The drawing under review shows one solid part. Ordinate dimensions are in mm from its lowest x, y, z. A direction names the side the tool comes from. Give positions to 0.01 mm unless a question says otherwise; leave off trailing zeros. Order: outer loops, then holes, each group sorted by start corner. A loop starts at its lowest first (then second) coordinate and runs counter-clockwise, first axis right, second up. Notation, with made-up numbers: (11.25, 24.5) -> (61.25, 24.5) arc R10 cw to (61.25, 40.5) -> close; hole circle Ø3 at (8.25, -24.5). An arc over 180 degrees is marked (long way). One line per item, written item: value. Start each with the question number.
1) Consider section C-C (z = 12). State the section outline as (x, y) points, plus the area to 3 significant figures.
2) Tool access review of the marked faces 1, 2 and 3: name each direction out of +Z, -Z, +X, -X, +Y, -Y from which nothing blocks a thin tool from reaching the whole face with its end or side.
3) The part is to be moulded in two halves that separate along Y. For the marked faces 4, 5, 6 and 7, say which applies: released by +Y, released by -Y, zero draft, split by the parting line, or undercut.
4) For pin 1 (5 mm diameter, centred on x = 8, y = 6, fed in from -Z); pin 2 (0.9 mm diameter, centred on x = 8.5, z = 4.5, fed in from +Y); pin 3 (1.5 mm diameter, centred on x = 7, y = 28, fed in from +Z), all flat-tipped, find the tip position at first contact; note any pin that passes through.
5) Consider section A-A (x = 10.5). State how many separate pieces and enclosed holes the cut face has, plus the area to 3 significant figures.
6) Wall thickness on line 1 along Z through (x, y) = (6, 14.9); line 2 along Z through (x, y) = (10.5, 24); line 3 along Y through (x, z) = (5.25, 3.5): over which ranges is each line inside the solid? List them lowest first. Write a range as from..to.
7) Consider section B-B (y = 14.9). State the section outline as (x, z) points.
8) Consider section D-D (y = 3.75). State the section outline as (x, z) points, plus the area to 3 significant figures.
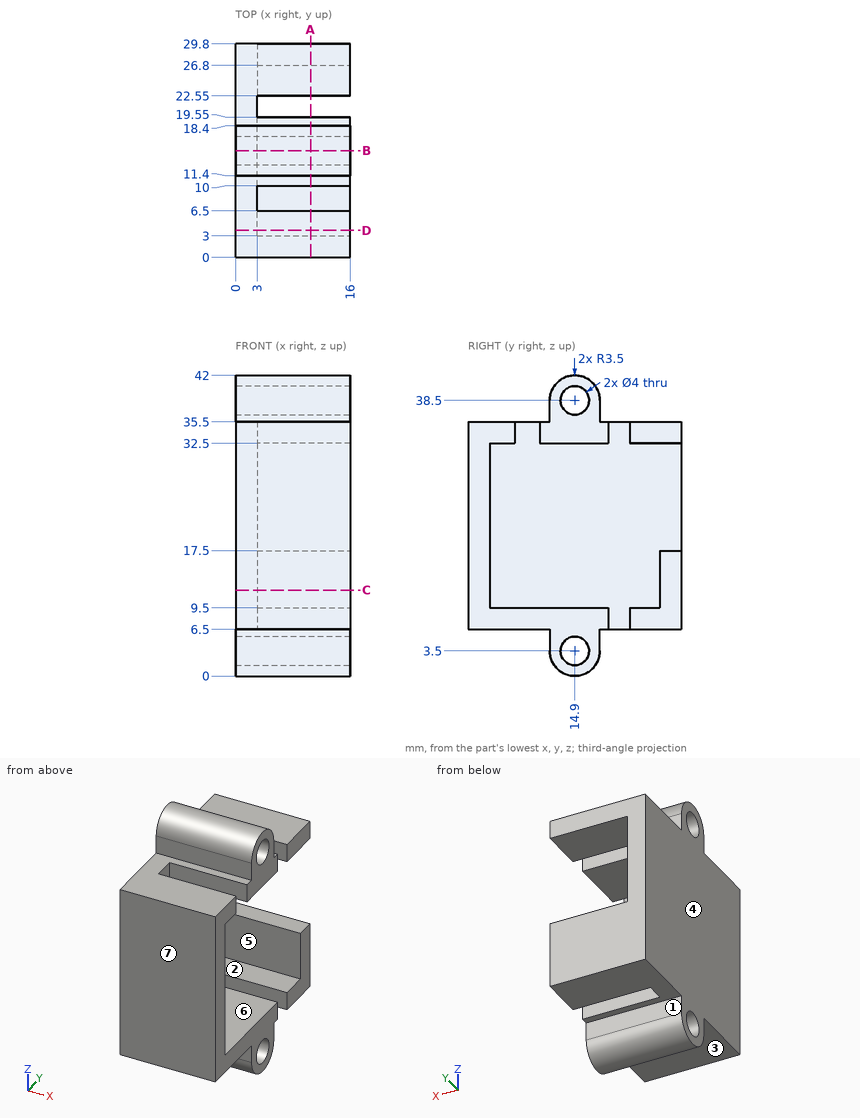
Checked values:
1. outline: (0, 0) -> (16, 0) -> (16, 3) -> (3, 3) -> (3, 26.8) -> (16, 26.8) -> (16, 29.8) -> (0, 29.8) -> close
1. area: 167 mm^2
2. face 1: -Z, +X, -X, +Y
2. face 2: +X
2. face 3: -Z, +X, -X, -Y
3. face 4: zero draft
3. face 5: undercut
3. face 6: undercut
3. face 7: released by -Y
4. pin 1: stops at z = 6.5
4. pin 2: stops at y = 18.4
4. pin 3: stops at z = 35.5
5. separate pieces: 4
5. enclosed holes: 2
5. area: 299 mm^2
6. line 1: z = 0..1.5, 5.5..9.5, 32.5..36.5, 40.5..42
6. line 2: z = 6.5..9.5, 32.5..35.5
6. line 3: y = 11.4..12.9, 16.9..18.4
7. outline: (0, 0) -> (16, 0) -> (16, 1.5) -> (0, 1.5) -> close; (0, 5.5) -> (16, 5.5) -> (16, 9.5) -> (3, 9.5) -> (3, 32.5) -> (16, 32.5) -> (16, 36.5) -> (0, 36.5) -> close; (0, 40.5) -> (16, 40.5) -> (16, 42) -> (0, 42) -> close
8. outline: (0, 6.5) -> (16, 6.5) -> (16, 9.5) -> (3, 9.5) -> (3, 32.5) -> (16, 32.5) -> (16, 35.5) -> (0, 35.5) -> close
8. area: 165 mm^2
